from build123d import *

# Parameters (mm, degrees)
SKETCH1_W               = 133.35
SKETCH1_H               = 0.65
SKETCH1_H_2             = 120
BOSS_EXTRUDE1_DEPTH     = 28.575
CUT_EXTRUDE2_DEPTH      = 141.221561288
CUT_EXTRUDE2_DEPTH_BACK = 141.221561288
SKETCH1_3_W             = 133.35
SKETCH1_3_H             = 0.65
SKETCH2_W               = 120
SKETCH2_H               = 7.15
CUT_EXTRUDE3_DEPTH      = 182.655589303
SKETCH3_R               = 35.56
CUT_EXTRUDE4_DEPTH      = 147.101182832
SKETCH4_W               = 42
SKETCH4_H               = 36.303073335
CUT_EXTRUDE5_DEPTH      = 147.101182832
M10_TAPPED_HOLE1_D      = 8.5
M10_TAPPED_HOLE1_DEPTH  = 27.5
M10_TAPPED_HOLE1_TIP    = 2.553657631
M12_TAPPED_HOLE1_D      = 10.2
M12_TAPPED_HOLE1_DEPTH  = 43.99
M12_TAPPED_HOLE1_TIP    = 3.064389157
CUT_EXTRUDE6_DEPTH      = 5.08
FILLET1_R               = 0.8128


with BuildPart() as part:
    # Sketch1 → Boss-Extrude1 (new, symmetric)
    with BuildSketch(Plane(origin=(0, 0, 0), x_dir=(1, 0, 0), z_dir=(0, 1, 0))):
        with Locations((0, -0.325)):
            Rectangle(SKETCH1_W, SKETCH1_H)
        with Locations((0, 60)):
            Rectangle(SKETCH1_W, SKETCH1_H_2)
    extrude(amount=BOSS_EXTRUDE1_DEPTH, both=True)

    # Sketch1_3 → Cut-Extrude2 (cut, two sides: drawn at the far end of the back side and taken through both)
    with BuildSketch(Plane(origin=(0, 0, 0), x_dir=(1, 0, 0), z_dir=(0, 1, 0)).offset(-CUT_EXTRUDE2_DEPTH_BACK)):
        with Locations((0, -0.325)):
            Rectangle(SKETCH1_3_W, SKETCH1_3_H)
    extrude(amount=CUT_EXTRUDE2_DEPTH + CUT_EXTRUDE2_DEPTH_BACK, mode=Mode.SUBTRACT)

    # Sketch2 → Cut-Extrude3 (cut, through all)
    with BuildSketch(Plane(origin=(66.675, 0, 0), x_dir=(0, 0, -1), z_dir=(1, 0, 0))):
        with Locations((60, 25)):
            Rectangle(SKETCH2_W, SKETCH2_H)
    extrude(amount=-CUT_EXTRUDE3_DEPTH, mode=Mode.SUBTRACT)

    # Sketch3 → Cut-Extrude4 (cut, through all)
    with BuildSketch(Plane(origin=(0, 21.425, 0), x_dir=(1, 0, 0), z_dir=(0, 1, 0))):
        with Locations(Location((0, 55, 0), (0, 0, 270))):
            Circle(SKETCH3_R)
    extrude(amount=-CUT_EXTRUDE4_DEPTH, mode=Mode.SUBTRACT)

    # Sketch4 → Cut-Extrude5 (cut, through all)
    with BuildSketch(Plane(origin=(0, 21.425, 0), x_dir=(1, 0, 0), z_dir=(0, 1, 0))):
        with Locations((0, 101.848463333)):
            Rectangle(SKETCH4_W, SKETCH4_H)
    extrude(amount=-CUT_EXTRUDE5_DEPTH, mode=Mode.SUBTRACT)

    # M10 Tapped Hole1
    with Locations(Plane(origin=(0, 21.425, 0), x_dir=(1, 0, 0), z_dir=(0, 1, 0))):
        with Locations((-38.97114317, 77.5), (-38.97114317, 32.5), (38.97114317, 77.5), (38.97114317, 32.5)):
            Hole(M10_TAPPED_HOLE1_D / 2, depth=M10_TAPPED_HOLE1_DEPTH)
            with Locations((0, 0, -(M10_TAPPED_HOLE1_DEPTH + M10_TAPPED_HOLE1_TIP / 2))):  # 118° drill point
                Cone(0, M10_TAPPED_HOLE1_D / 2, M10_TAPPED_HOLE1_TIP, mode=Mode.SUBTRACT)

    # M12 Tapped Hole1
    with Locations(Plane.XY):
        with Locations((-53, 9.425), (-53, -14.575), (53, 9.425), (53, -14.575)):
            Hole(M12_TAPPED_HOLE1_D / 2, depth=M12_TAPPED_HOLE1_DEPTH)
            with Locations((0, 0, -(M12_TAPPED_HOLE1_DEPTH + M12_TAPPED_HOLE1_TIP / 2))):  # 118° drill point
                Cone(0, M12_TAPPED_HOLE1_D / 2, M12_TAPPED_HOLE1_TIP, mode=Mode.SUBTRACT)

    # Sketch9 → Cut-Extrude6 (cut)
    with BuildSketch(Plane.XY):
        with BuildLine():
            Line((-25.4, 3.425), (25.4, 3.425))
            ThreePointArc((25.4, 3.425), (31.4, -2.575), (25.4, -8.575))
            Line((25.4, -8.575), (-25.4, -8.575))
            ThreePointArc((-25.4, -8.575), (-31.4, -2.575), (-25.4, 3.425))
        make_face()
    extrude(amount=-CUT_EXTRUDE6_DEPTH, mode=Mode.SUBTRACT)

    # Fillet1
    fillet1_edges = [part.edges().sort_by_distance(p)[0] for p in [
        (-31.4, -2.575, -5.08),
        (0, 3.425, -5.08),
        (31.4, -2.575, -5.08),
        (0, -8.575, -5.08),
    ]]
    fillet(fillet1_edges, radius=FILLET1_R)


solid = part.part
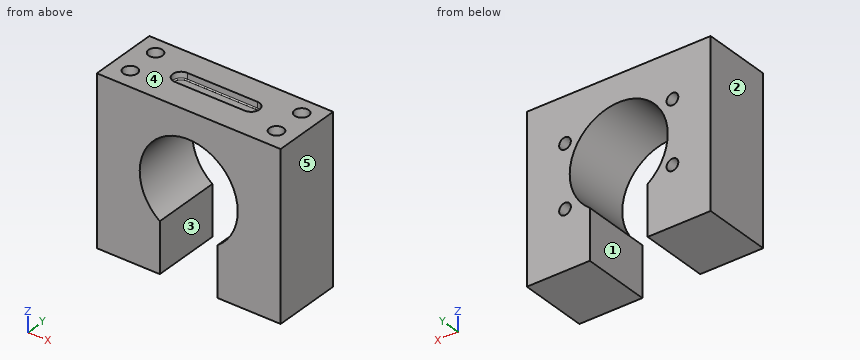
Could you check a few things on this model? Use its own coordinates, in mm. Face numbers are marked on the shaded views. A direction names the side the tool comes from. Give positions to 0.01 mm unless a question says otherwise; leave off trailing zeros. Write each loop counter-clockwise with the first axis right and the second up, starting at its lowest first coordinate (ties: lowest second). Pieces come first, ordered by that corner, then holes. Notation, with made-up numbers: (17, -30) -> (51, -30) arc R16 ccw to (51, -15) -> close; hole circle Ø7 at (59, 77.5). An arc over 180 degrees is marked (long way). Write each question's results on one line, items separated by ' | '. Start each with the question number.
Q1. Suppose I cut it at D-D, the plane z = -34.5. State how many separate pieces and enclosed holes the cut face has, and give its area (3 significant figures).
Q2. I'm going to push flat-ended pins straight in: pin 1 Ø8.5 at (x, y) = (0.5, -3) entering from +Z; pin 2 Ø7.5 at (x, z) = (-38.97, -32.5) entering from +Y; pin 3 Ø7 at (x, z) = (-38.97, -77.5) entering from +Y. Where does each tip first touch, or does it pass through?
Q3. Which directions (+Z, -Z, +X, -X, +Y, -Y) give clear straight access to the entire face, cutting with the end or side of a thin tool? Please do the marked faces 1 and 2.
Q4. Suppose I cut it at C-C, the plane x = 0. List the corners of the cut face in (y, z) for me (3 decimals).
Q5. I need wall thicknesses on probe 1 along Y at (x, z) = (53, -21) (3 decimals); probe 2 along X at (y, z) = (-9, -86) (3 decimals); probe 3 along Z at (x, y) = (-40.5, -5.5). Which ranges of each line are inside material? Lowest first, please.
Q6. Suppose I cut it at A-A, the plane z = -55. List the corners of the cut face in (x, y) for me (3 decimals).
Q7. We'd pull the mould along X, two halves only. Please class the marked faces 3, 4 and 5: +X half, -X half, draft (parallel to the pull), parting line (faces both ways), or undercut.
Q8. Suppose I cut it at B-B, the plane z = -99. List the corners of the cut face in (x, y) for me (3 decimals).
Outcome:
1) separate pieces: 2 | enclosed holes: 4 | area: 3,010 mm2
2) pin 1: z = -5.08 | pin 2: y = -6.37 | pin 3: y = -6.52
3) face 1: -Z, +Y, -Y | face 2: +Z, -Z, -X, +Y, -Y
4) outline: (-28.575, -19.44) -> (21.425, -19.44) -> (21.425, 0) -> (3.425, 0) -> (3.425, -4.267) arc R0.813 cw to (2.612, -5.08) -> (-7.762, -5.08) arc R0.813 cw to (-8.575, -4.267) -> (-8.575, 0) -> (-28.575, 0) -> close
5) probe 1: -28.575 to -19.675, -9.475 to 4.325, 14.525 to 21.425 | probe 2: -66.675 to -21, 21 to 66.675 | probe 3: -120 to -81.47, -73.53 to -36.47, -28.53 to 0
6) outline: (-66.675, -28.575) -> (-35.56, -28.575) -> (-35.56, 21.425) -> (-66.675, 21.425) -> close; (35.56, -28.575) -> (66.675, -28.575) -> (66.675, 21.425) -> (35.56, 21.425) -> close
7) face 3: undercut | face 4: draft | face 5: +X half
8) outline: (-66.675, -28.575) -> (-21, -28.575) -> (-21, 21.425) -> (-66.675, 21.425) -> close; (21, -28.575) -> (66.675, -28.575) -> (66.675, 21.425) -> (21, 21.425) -> close
